Work out the finished part from the listing and answer in its coordinate system (mm). A direction names the side the tool comes from. Round coordinates to 2 decimals unless told otherwise and drop trailing zeros. Write each loop counter-clockwise with the first axis right and the second up, starting at its lowest first coordinate (ties: lowest second). Pieces come first, ordered by that corner, then holes. Notation, with made-up numbers: (77.25, -20.75) -> (104.25, -20.75) arc R9 ccw to (104.25, -13.75) -> close; hole circle Ø6 at (18.25, 53.5). An arc over 180 degrees is marked (long way). Answer as a JSON object with one key per item and string values. Group by question number.
from build123d import *

# Parameters (mm, degrees)
F1_DEPTH = 11.1125
F2_DEPTH = 60.325
F0_W     = 11.1125
F0_H     = 33.3375
F3_DEPTH = 50.8
F6_DEPTH = 11.1125
F7_DEPTH = 11.1125
F4_R     = 7.9375
F8_DEPTH = 11.1125


# Not quite as in the source:
# - a length typed as a fraction of an inch, garbled in the dataset ("3 / 203.2 mm" for 3/8 in), is restored


with BuildPart() as f1:
    # F0 (on Top) → F1 (new body)
    with BuildSketch(Plane.XY):
        Polygon((-46.0375, 11.1125), (-46.0375, -22.225), (6.35, 11.1125), (-25.4, 11.1125), align=None)
    extrude(amount=F1_DEPTH)

    # F0 (on Top) → F2 (join)
    with BuildSketch(Plane.XY):
        Polygon((-57.15, 11.1125), (-46.0375, 11.1125), (-25.4, 11.1125), (-25.4, 22.225), (-57.15, 22.225), align=None)
        Polygon((-25.4, 11.1125), (6.35, 11.1125), (57.15, 11.1125), (57.15, 22.225), (-25.4, 22.225), align=None)
    extrude(amount=F2_DEPTH)

    # F0 (on Top) → F3 (join)
    with BuildSketch(Plane.XY):
        with Locations((-51.59375, -5.55625)):
            Rectangle(F0_W, F0_H)
    extrude(amount=F3_DEPTH)

    # F5 (on face) → F6 (cut)
    with BuildSketch(Plane.YZ.offset(-46.0375)):
        Polygon((-22.225, 50.8), (-22.225, 21.9288781013), (-5.55625, 50.8), align=None)
    extrude(amount=-F6_DEPTH, mode=Mode.SUBTRACT)

    # F4 (on face) → F7 (cut)
    with BuildSketch(Plane.XZ.offset(-11.1125)):
        Polygon((57.15, 60.325), (-25.4, 60.325), (57.15, 38.2057941648), align=None)
    extrude(amount=-F7_DEPTH, mode=Mode.SUBTRACT)

    # F4 (on face) → F8 (cut)
    with BuildSketch(Plane.XZ.offset(-11.1125)):
        with Locations((38.1, 19.05)):
            Circle(F4_R)
    extrude(amount=-F8_DEPTH, mode=Mode.SUBTRACT)


solid = f1.part
1) Each of these flat-tipped pins is pushed along its axis until it touches: P1, Ø5, axis at x = -0.5, z = 49, coming from the -Y side; P2, Ø4, axis at y = 6.5, z = 52.5, coming from the +X side; P3, Ø5, axis at x = -45, y = -7.5, coming from the +Z side; P4, Ø10, axis at y = 6, z = 52.5, coming from the -X side. Where does it stop, or does it pass through?
2) A tool of negligible diameter and unlimited length cuts with its end or side. For faces 1 (the face through (-20.21, -5.79, 5.48)), 2 (the face through (-46.038, -2, 31)), 3 (the face through (-52, 3, 50.8)), from which of +Z, -Z, +X, -X, +Y, -Y can it reach the whole face along a straight path? Write none if from no direction.
3) For a pull along Z with two mould halves and no side action, classify faces 4 (the face through (1, 22.225, 30)), 5 (the face through (31.8, 16.59, 14.22)), 6 (the face through (-26, -2, 11.112)), 7 (the face through (-14, 5, 0)) as released by +Z, released by -Z, zero draft, split by the parting line, or undercut.
4) A cutting plane is placed at C-C on x = 38.1. Determine the outline of the cut face in (y, z) (1 decimal).
5) Straight lines are drawn through the part: L1, parallel to X at y = 18, z = 19; L2, parallel to Z at x = -44.5, y = -2; L3, parallel to Y at x = -19, z = 32.5 (1 decimal). For each, find the intervals that lie inside material, in ascending order.
6) A cutting plane is placed at D-D on x = -19. Determine the outline of the cut face in (y, z) (1 decimal), plus the area to 3 significant figures.
Established:
{
 "1": {"P1": "stops at y = 11.11", "P2": "stops at x = -46.04", "P3": "stops at z = 50.8", "P4": "stops at x = -57.15"},
 "2": {"face 1": "+Z, -Z, +X, -Y", "face 2": "+Z, +X, -Y", "face 3": "+Z, +X, -X, -Y"},
 "3": {"face 4": "zero draft", "face 5": "undercut", "face 6": "released by +Z", "face 7": "released by -Z"},
 "4": {"outline": "(11.1, 0) -> (22.2, 0) -> (22.2, 11.1) -> (11.1, 11.1) -> close; (11.1, 27) -> (22.2, 27) -> (22.2, 43.3) -> (11.1, 43.3) -> close"},
 "5": {"L1": "x = -57.15 to 30.16, 46.04 to 57.15", "L2": "z = 0 to 11.11", "L3": "y = 11.1 to 22.2"},
 "6": {"outline": "(-5, 0) -> (22.2, 0) -> (22.2, 58.6) -> (11.1, 58.6) -> (11.1, 11.1) -> (-5, 11.1) -> close", "area": "831 mm²"}
}
